Work out the finished part from the listing and answer in its coordinate system (mm). Coordinates: 2 decimals unless noted, no trailing zeros. Order: outer loops, then holes, each group sorted by start corner. A loop starts at its lowest first (then second) coordinate and runs counter-clockwise, first axis right, second up.
1. The part is cut by section C-C, the plane x = 78.74. Give the vertices of the cut face in (y, z), then the cut area to 3 significant figures.
2. Find the intervals of material crossed by probe 1 along X at (y, z) = (0.2, 0); probe 2 along Z at (x, y) = (78.74, 0.1); probe 3 along Z at (x, y) = (-77, 0.1), in increasing order.
3. A flat-ended cylindrical pin translates along its axis: pin 1 Ø4 at (x, z) = (78.74, 0) entering from +Y. Find the tip coordinate at first contact, or state that the pin passes through.
4. The part is cut by section A-A, the plane z = 0. Give the vertices of the cut face in (x, y).
5. The part is cut by section B-B, the plane x = 0. Give the vertices of the cut face in (y, z) (3 decimals), then the cut area to 3 significant figures.
```python
from build123d import *

# Parameters (mm, degrees)
SKETCH1_W           = 172.72
SKETCH1_H           = 52.07
BOSS_EXTRUDE1_DEPTH = 0.25
FILLET1_R           = 10
SKETCH2_R           = 1.6
CUT_EXTRUDE1_DEPTH  = 91.199408673


with BuildPart() as part:
    # Sketch1 → Boss-Extrude1 (new body)
    with BuildSketch(Plane(origin=(0, 0, 0), x_dir=(1, 0, 0), z_dir=(0, 1, 0))):
        Rectangle(SKETCH1_W, SKETCH1_H)
    extrude(amount=BOSS_EXTRUDE1_DEPTH)

    # Fillet1
    fillet1_edges = [part.edges().sort_by_distance(p)[0] for p in [
        (86.36, 0.125, 26.035),
        (-86.36, 0.125, 26.035),
        (-86.36, 0.125, -26.035),
        (86.36, 0.125, -26.035),
    ]]
    fillet(fillet1_edges, radius=FILLET1_R)

    # Sketch2 → Cut-Extrude1 (cut, through all)
    with BuildSketch(Plane(origin=(0, 0.25, 0), x_dir=(1, 0, 0), z_dir=(0, 1, 0))):
        with Locations(Location((-78.74, 0, 0), (0, 0, 270))):
            Circle(SKETCH2_R)
        with Locations(Location((0, 0, 0), (0, 0, 270))):
            Circle(SKETCH2_R)
    cut_extrude1 = extrude(amount=-CUT_EXTRUDE1_DEPTH, mode=Mode.SUBTRACT)

    # Mirror1: Cut-Extrude1 across plane
    add(cut_extrude1.mirror(Plane(origin=(0, 0, 0), x_dir=(0, 0, 1), z_dir=(1, 0, 0))), mode=Mode.SUBTRACT)


solid = part.part
```
Geometry says:
1. outline: (0, -25.75) - (0.25, -25.75) - (0.25, -1.6) - (0, -1.6) - close; (0, 1.6) - (0.25, 1.6) - (0.25, 25.75) - (0, 25.75) - close
1. area: 12.1 mm2
2. probe 1: x = -86.36 to -80.34, -77.14 to -1.6, 1.6 to 77.14, 80.34 to 86.36
2. probe 2: z = -25.75 to -1.6, 1.6 to 25.75
2. probe 3: z = -26.01 to 26.01
3. pin 1: stops at y = 0.25
4. outline: (-86.36, 0) - (-80.34, 0) - (-80.34, 0.25) - (-86.36, 0.25) - close; (-77.14, 0) - (-1.6, 0) - (-1.6, 0.25) - (-77.14, 0.25) - close; (1.6, 0) - (77.14, 0) - (77.14, 0.25) - (1.6, 0.25) - close; (80.34, 0) - (86.36, 0) - (86.36, 0.25) - (80.34, 0.25) - close
5. outline: (0, -26.035) - (0.25, -26.035) - (0.25, -1.6) - (0, -1.6) - close; (0, 1.6) - (0.25, 1.6) - (0.25, 26.035) - (0, 26.035) - close
5. area: 12.2 mm2
